```python
from build123d import *

# Parameters (mm, degrees)
EXTRUDE_1_DEPTH     = 17
SKETCH_5_R          = 3
CUT_EXTRUDE_3_DEPTH = 49
SKETCH_6_W          = 49
SKETCH_6_H          = 4
EXTRUDE_3_DEPTH     = 50
SKETCH_7_W          = 67
SKETCH_7_H          = 4
EXTRUDE_4_DEPTH     = 18.5
SKETCH_8_W          = 67
SKETCH_8_H          = 4
EXTRUDE_5_DEPTH     = 18.5
SKETCH_14_W         = 49
SKETCH_14_H         = 4
EXTRUDE_13_DEPTH    = 66
SKETCH_23_W         = 49
SKETCH_23_H         = 19.9
EXTRUDE_18_DEPTH    = 17
CUT_EXTRUDE_4_REACH = 6
SKETCH_13_R         = 2.05
EXTRUDE_14_DEPTH    = 5
EXTRUDE_15_DEPTH    = 5
CUT_EXTRUDE_5_REACH = 23
SKETCH_18_R         = 2.1
SKETCH_21_W         = 34.5
SKETCH_21_H         = 0.7
CUT_EXTRUDE_6_DEPTH = 4.6
EXTRUDE_19_DEPTH    = 3
EXTRUDE_20_DEPTH    = 3
EXTRUDE_21_REACH    = 42
SKETCH_29_W         = 4.15
SKETCH_29_H         = 17
SKETCH_29_W_2       = 4.65
SKETCH_3_W          = 2
SKETCH_3_H          = 12.5
CUT_EXTRUDE_7_DEPTH = 17
CUT_EXTRUDE_8_DEPTH = 20


with BuildPart() as part:
    # Эскиз1 → Бобышка-Вытянуть1 (new body)
    with BuildSketch(Plane.XY):
        Polygon((-13.125, 2.698768931), (-15.5, 2.698768931), (-15.5, 4.138768931), (-12.84, 6.798768931), (-7.36, 6.798768931), (-4.7, 4.138768931), (-4.7, 2.698768931), (-7.075, 2.698768931), (-7.075, 0.698768931), (6.875, 0.698768931), (6.875, 2.698768931), (4.5, 2.698768931), (4.5, 4.138768931), (7.16, 6.798768931), (12.64, 6.798768931), (15.3, 4.138768931), (15.3, 2.698768931), (12.925, 2.698768931), (12.925, 0.698768931), (24.65, 0.698768931), (24.65, -29.301231069), (15.25, -29.301231069), (15.25, -4.901231069), (-19.45, -4.901231069), (-19.45, -29.301231069), (-24.35, -29.301231069), (-24.35, 0.698768931), (-13.125, 0.698768931), align=None)
    extrude(amount=EXTRUDE_1_DEPTH)

    # Эскиз5 → Вырез-Вытянуть3 (cut)
    with BuildSketch(Plane.ZY.offset(24.35)):
        with Locations((9, -17.301231069)):
            Circle(SKETCH_5_R)
    extrude(amount=-CUT_EXTRUDE_3_DEPTH, mode=Mode.SUBTRACT)

    # Эскиз6 → Бобышка-Вытянуть3 (add)
    with BuildSketch(Plane.XY.offset(17)):
        with Locations((0.15, -27.301231069)):
            Rectangle(SKETCH_6_W, SKETCH_6_H)
    extrude(amount=EXTRUDE_3_DEPTH)

    # Эскиз7 → Бобышка-Вытянуть4 (add)
    with BuildSketch(Plane.ZY.offset(24.35)):
        with Locations((33.5, -27.301231069)):
            Rectangle(SKETCH_7_W, SKETCH_7_H)
    extrude(amount=EXTRUDE_4_DEPTH)

    # Эскиз8 → Бобышка-Вытянуть5 (add)
    with BuildSketch(Plane(origin=(24.65, 0, 0), x_dir=(0, 0, -1), z_dir=(1, 0, 0))):
        with Locations((-33.5, -27.301231069)):
            Rectangle(SKETCH_8_W, SKETCH_8_H)
    extrude(amount=EXTRUDE_5_DEPTH)

    # Эскиз14 → Бобышка-Вытянуть13 (add)
    with BuildSketch(Plane(origin=(0, -25.301231069, 0), x_dir=(1, 0, 0), z_dir=(0, 1, 0))):
        with Locations((0.15, -19)):
            Rectangle(SKETCH_14_W, SKETCH_14_H)
    extrude(amount=EXTRUDE_13_DEPTH)

    # Эскиз23 → Бобышка-Вытянуть18 (add)
    with BuildSketch(Plane(origin=(0, 0, 17), x_dir=(-1, 0, 0), z_dir=(0, 0, -1))):
        with Locations((-0.15, 30.748768931)):
            Rectangle(SKETCH_23_W, SKETCH_23_H)
    extrude(amount=EXTRUDE_18_DEPTH)

    # Эскиз13 → Вырез-Вытянуть4 (cut, up to next)
    with BuildSketch(Plane(origin=(0, -25.301231069, 0), x_dir=(1, 0, 0), z_dir=(0, 1, 0)), mode=Mode.PRIVATE) as cut_extrude_4_sk1:
        with Locations((-8.85, -58)):
            Circle(SKETCH_13_R)
    cut_extrude_4_tool1 = extrude(cut_extrude_4_sk1.sketch, amount=-CUT_EXTRUDE_4_REACH, mode=Mode.PRIVATE) & part.part
    add(cut_extrude_4_tool1.solids().sort_by_distance((-8.85, -25.301231, 58))[0], mode=Mode.SUBTRACT)
    # Эскиз13 → Вырез-Вытянуть4 (cut, up to next)
    with BuildSketch(Plane(origin=(0, -25.301231069, 0), x_dir=(1, 0, 0), z_dir=(0, 1, 0)), mode=Mode.PRIVATE) as cut_extrude_4_sk2:
        with Locations((9.15, -58)):
            Circle(SKETCH_13_R)
    cut_extrude_4_tool2 = extrude(cut_extrude_4_sk2.sketch, amount=-CUT_EXTRUDE_4_REACH, mode=Mode.PRIVATE) & part.part
    add(cut_extrude_4_tool2.solids().sort_by_distance((9.15, -25.301231, 58))[0], mode=Mode.SUBTRACT)
    # Эскиз13 → Вырез-Вытянуть4 (cut, up to next)
    with BuildSketch(Plane(origin=(0, -25.301231069, 0), x_dir=(1, 0, 0), z_dir=(0, 1, 0)), mode=Mode.PRIVATE) as cut_extrude_4_sk3:
        with Locations((-33.85, -11)):
            Circle(SKETCH_13_R)
    cut_extrude_4_tool3 = extrude(cut_extrude_4_sk3.sketch, amount=-CUT_EXTRUDE_4_REACH, mode=Mode.PRIVATE) & part.part
    add(cut_extrude_4_tool3.solids().sort_by_distance((-33.85, -25.301231, 11))[0], mode=Mode.SUBTRACT)
    # Эскиз13 → Вырез-Вытянуть4 (cut, up to next)
    with BuildSketch(Plane(origin=(0, -25.301231069, 0), x_dir=(1, 0, 0), z_dir=(0, 1, 0)), mode=Mode.PRIVATE) as cut_extrude_4_sk4:
        with Locations((34.15, -11)):
            Circle(SKETCH_13_R)
    cut_extrude_4_tool4 = extrude(cut_extrude_4_sk4.sketch, amount=-CUT_EXTRUDE_4_REACH, mode=Mode.PRIVATE) & part.part
    add(cut_extrude_4_tool4.solids().sort_by_distance((34.15, -25.301231, 11))[0], mode=Mode.SUBTRACT)
    # Эскиз13 → Вырез-Вытянуть4 (cut, up to next)
    with BuildSketch(Plane(origin=(0, -25.301231069, 0), x_dir=(1, 0, 0), z_dir=(0, 1, 0)), mode=Mode.PRIVATE) as cut_extrude_4_sk5:
        with Locations((-8.85, -30)):
            Circle(SKETCH_13_R)
    cut_extrude_4_tool5 = extrude(cut_extrude_4_sk5.sketch, amount=-CUT_EXTRUDE_4_REACH, mode=Mode.PRIVATE) & part.part
    add(cut_extrude_4_tool5.solids().sort_by_distance((-8.85, -25.301231, 30))[0], mode=Mode.SUBTRACT)
    # Эскиз13 → Вырез-Вытянуть4 (cut, up to next)
    with BuildSketch(Plane(origin=(0, -25.301231069, 0), x_dir=(1, 0, 0), z_dir=(0, 1, 0)), mode=Mode.PRIVATE) as cut_extrude_4_sk6:
        with Locations((9.15, -30)):
            Circle(SKETCH_13_R)
    cut_extrude_4_tool6 = extrude(cut_extrude_4_sk6.sketch, amount=-CUT_EXTRUDE_4_REACH, mode=Mode.PRIVATE) & part.part
    add(cut_extrude_4_tool6.solids().sort_by_distance((9.15, -25.301231, 30))[0], mode=Mode.SUBTRACT)

    # Эскиз16 → Бобышка-Вытянуть14 (add)
    with BuildSketch(Plane.ZY.offset(24.35)):
        Polygon((21, -25.301231069), (21, 40.698768931), (67, -25.301231069), align=None)
    extrude(amount=-EXTRUDE_14_DEPTH)

    # Эскиз17 → Бобышка-Вытянуть15 (add)
    with BuildSketch(Plane(origin=(24.65, 0, 0), x_dir=(0, 0, -1), z_dir=(1, 0, 0))):
        Polygon((-67, -25.301231069), (-21, 40.698768931), (-21, -25.301231069), align=None)
    extrude(amount=-EXTRUDE_15_DEPTH)

    # Эскиз18 → Вырез-Вытянуть5 (cut, up to next)
    with BuildSketch(Plane.XY.offset(21), mode=Mode.PRIVATE) as cut_extrude_5_sk1:
        with Locations((9.85, 10.798768931)):
            Circle(SKETCH_18_R)
    cut_extrude_5_tool1 = extrude(cut_extrude_5_sk1.sketch, amount=-CUT_EXTRUDE_5_REACH, mode=Mode.PRIVATE) & part.part
    add(cut_extrude_5_tool1.solids().sort_by_distance((9.85, 10.798769, 21))[0], mode=Mode.SUBTRACT)
    # Эскиз18 → Вырез-Вытянуть5 (cut, up to next)
    with BuildSketch(Plane.XY.offset(21), mode=Mode.PRIVATE) as cut_extrude_5_sk2:
        with Locations((-10.15, 10.798768931)):
            Circle(SKETCH_18_R)
    cut_extrude_5_tool2 = extrude(cut_extrude_5_sk2.sketch, amount=-CUT_EXTRUDE_5_REACH, mode=Mode.PRIVATE) & part.part
    add(cut_extrude_5_tool2.solids().sort_by_distance((-10.15, 10.798769, 21))[0], mode=Mode.SUBTRACT)

    # Эскиз21 → Вырез-Вытянуть6 (cut)
    with BuildSketch(Plane(origin=(0, 0, 0), x_dir=(-1, 0, 0), z_dir=(0, 0, -1))):
        with Locations((2, -4.551231069)):
            Rectangle(SKETCH_21_W, SKETCH_21_H)
    extrude(amount=-CUT_EXTRUDE_6_DEPTH, mode=Mode.SUBTRACT)

    # Эскиз25 → Бобышка-Вытянуть19 (add)
    with BuildSketch(Plane(origin=(0, 0, 0), x_dir=(-1, 0, 0), z_dir=(0, 0, -1))):
        Polygon((-24.65, 40.698768931), (-24.65, -25.301231069), (-43.15, -25.301231069), align=None)
        Polygon((42.85, -25.301231069), (24.35, -25.301231069), (24.35, 40.698768931), align=None)
    extrude(amount=-EXTRUDE_19_DEPTH)

    # Эскиз28 → Бобышка-Вытянуть20 (add)
    with BuildSketch(Plane.XY.offset(21)):
        Polygon((43.15, -25.301231069), (24.65, -25.301231069), (24.65, 40.698768931), align=None)
        Polygon((-24.35, -25.301231069), (-42.85, -25.301231069), (-24.35, 40.698768931), align=None)
    extrude(amount=-EXTRUDE_20_DEPTH)

    # Эскиз29 → Бобышка-Вытянуть21 (add, up to next)
    with BuildSketch(Plane(origin=(0, 0.698768931, 0), x_dir=(1, 0, 0), z_dir=(0, 1, 0)), mode=Mode.PRIVATE) as extrude_21_sk1:
        with Locations((-22.275, -8.5)):
            Rectangle(SKETCH_29_W, SKETCH_29_H)
    extrude_21_tool1 = extrude(extrude_21_sk1.sketch, amount=EXTRUDE_21_REACH, mode=Mode.PRIVATE) - part.part
    add(extrude_21_tool1.solids().sort_by_distance((-22.275, 0.698769, 8.5))[0])
    # Эскиз29 → Бобышка-Вытянуть21 (add, up to next)
    with BuildSketch(Plane(origin=(0, 0.698768931, 0), x_dir=(1, 0, 0), z_dir=(0, 1, 0)), mode=Mode.PRIVATE) as extrude_21_sk2:
        with Locations((22.325, -8.5)):
            Rectangle(SKETCH_29_W_2, SKETCH_29_H)
    extrude_21_tool2 = extrude(extrude_21_sk2.sketch, amount=EXTRUDE_21_REACH, mode=Mode.PRIVATE) - part.part
    add(extrude_21_tool2.solids().sort_by_distance((22.325, 0.698769, 8.5))[0])

    # Эскиз3 → Вырез-Вытянуть7 (cut)
    with BuildSketch(Plane(origin=(0, 0, 0), x_dir=(-1, 0, 0), z_dir=(0, 0, -1))):
        with Locations((20.25, -17.051231069)):
            Rectangle(SKETCH_3_W, SKETCH_3_H)
    extrude(amount=-CUT_EXTRUDE_7_DEPTH, mode=Mode.SUBTRACT)

    # Эскиз30 → Вырез-Вытянуть8 (cut)
    with BuildSketch(Plane(origin=(0, 40.698768931, 0), x_dir=(1, 0, 0), z_dir=(0, 1, 0))):
        Polygon((-4.2, 0), (4, 0), (4, -1.4), (8.1, -3.4), (8.1, -4.6), (4, -6.6), (-4.2, -6.6), (-8.3, -4.6), (-8.3, -3.4), (-4.2, -1.4), align=None)
    extrude(amount=-CUT_EXTRUDE_8_DEPTH, mode=Mode.SUBTRACT)


solid = part.part
```
Input: part model. Units: mm. Frame: model coordinates. A direction names the side the tool comes from. Give positions to 0.01 mm unless a question says otherwise; leave off trailing zeros. Order: outer loops, then holes, each group sorted by start corner. A loop starts at its lowest first (then second) coordinate and runs counter-clockwise, first axis right, second up. Notation, with made-up numbers: (-13, 78) - (9, 78) arc R28 cw to (9, 96) - close; hole circle Ø7 at (-9, 0). An arc over 180 degrees is marked (long way). Use a Markdown table: item, result.
(1) Section query B-B (x = -33.85). Output: boundary loops of the cut face in (y, z).
Computed values:
| item | result |
|---|---|
| outline | (-29.3, 0) - (6.81, 0) - (6.81, 3) - (-25.3, 3) - (-25.3, 8.95) - (-29.3, 8.95) - close; (-29.3, 13.05) - (-25.3, 13.05) - (-25.3, 18) - (6.81, 18) - (6.81, 21) - (-25.3, 21) - (-25.3, 67) - (-29.3, 67) - close |
(2) Draft query along X for faces 1 (the flat face through (33.77, 8.16, 19.52)), 2 (the flat face through (20, 11, 9)), 3 (the flat face through (0, -29.301, 34)), 4 (the flat face through (-2, -4.201, 2)). Return one class per face: released by +X, released by -X, zero draft, split by the parting line, or undercut.
Computed values:
| item | result |
|---|---|
| face 1 | released by +X |
| face 2 | undercut |
| face 3 | zero draft |
| face 4 | undercut |
(3) Access query for faces 5 (the flat face through (24.65, 8, 10)), 6 (the flat face through (43.15, -27, 34)), 7 (the cylindrical face through (8.883, -27.273, 55.967)), 8 (the flat face through (15.25, -14, 8)), 9 (the flat face through (14, 2.699, 8)). Directions: +Z, -Z, +X, -X, +Y, -Y. A direction counts if a zero-diameter tool reaches every point of the face in a straight line with its end or side. Return the directions, or none.
Computed values:
| item | result |
|---|---|
| face 5 | +X, +Y |
| face 6 | +Z, -Z, +X, +Y, -Y |
| face 7 | +Y, -Y |
| face 8 | -Z, -Y |
| face 9 | -Z |
(4) Section query C-C (z = 23). Output: boundary loops of the cut face in (x, y).
Computed values:
| item | result |
|---|---|
| outline | (-42.85, -29.3) - (43.15, -29.3) - (43.15, -25.3) - (24.65, -25.3) - (24.65, 37.83) - (19.65, 37.83) - (19.65, -25.3) - (-19.35, -25.3) - (-19.35, 37.83) - (-24.35, 37.83) - (-24.35, -25.3) - (-42.85, -25.3) - close |
(5) Section query D-D (x = -17.5). Output: boundary loops of the cut face in (y, z), then the cut area to 3 significant figures.
Computed values:
| item | result |
|---|---|
| outline | (-29.3, 17) - (-4.9, 17) - (-4.9, 4.6) - (-4.2, 4.6) - (-4.2, 0) - (0.7, 0) - (0.7, 17) - (20.8, 17) - (20.8, 0) - (40.7, 0) - (40.7, 21) - (-25.3, 21) - (-25.3, 67) - (-29.3, 67) - close |
| area | 894 mm2 |
(6) Pin query (flat end, axial travel): pin 1 (15 mm diameter, centred on x = 33.5, y = 7, fed in from +Z); pin 2 (0.7 mm diameter, centred on y = 3.5, z = 5, fed in from -X); pin 3 (1 mm diameter, centred on x = 33.5, z = 50, fed in from +Y); pin 4 (3 mm diameter, centred on x = 19.5, y = 14, fed in from -Z). Return the tip coordinate at first contact, or that it passes through.
Computed values:
| item | result |
|---|---|
| pin 1 | stops at z = 21 |
| pin 2 | stops at x = -24.35 |
| pin 3 | stops at y = -25.3 |
| pin 4 | stops at z = 0 |
(7) Line query: line 1 (X direction, y = -28.4, z = 11); line 2 (Y direction, x = 18, z = 9); line 3 (X direction, y = -3, z = 48.5). Output: solid intervals per line, ascending. Write a range as from..to.
Computed values:
| item | result |
|---|---|
| line 1 | x = -42.85..-35.9, -31.8..-19.45, 15.25..32.1, 36.2..43.15 |
| line 2 | y = -29.3..-20.3, -14.3..0.7, 20.8..40.7 |
| line 3 | x = -24.35..-19.35, 19.65..24.65 |
(8) Section query A-A (x = 9.85). Output: boundary loops of the cut face in (y, z).
Computed values:
| item | result |
|---|---|
| outline | (-29.3, 17) - (-4.9, 17) - (-4.9, 4.6) - (-4.2, 4.6) - (-4.2, 0) - (6.8, 0) - (6.8, 17) - (8.7, 17) - (8.7, 21) - (-25.3, 21) - (-25.3, 28.07) - (-29.3, 28.07) - close; (-29.3, 31.93) - (-25.3, 31.93) - (-25.3, 56.07) - (-29.3, 56.07) - close; (-29.3, 59.93) - (-25.3, 59.93) - (-25.3, 67) - (-29.3, 67) - close; (12.9, 17) - (20.8, 17) - (20.8, 0) - (40.7, 0) - (40.7, 21) - (12.9, 21) - close |
